from build123d import *

# Parameters (mm, degrees)
SALIENTE_EXTRUIR1_DEPTH = 155
CORTAR_EXTRUIR6_DEPTH   = 155
CROQUIS5_R              = 1.5
CORTAR_EXTRUIR9_DEPTH   = 155


with BuildPart() as part:
    # Croquis1 → Saliente-Extruir1 (new body)
    with BuildSketch(Plane.XY):
        with BuildLine():
            Line((0, 0), (28.5, 0))
            Line((28.5, 0), (0, 3))
            ThreePointArc((0, 3), (-1.5, 1.5), (0, 0))
        make_face()
    extrude(amount=-SALIENTE_EXTRUIR1_DEPTH)

    # Croquis3 → Cortar-Extruir6 (cut)
    with BuildSketch(Plane(origin=(0, 0, 0), x_dir=(1, 0, 0), z_dir=(0, 1, 0))):
        Polygon((28.5, 0), (28.5, 117.287187079), (16.5, 0), align=None)
        with BuildLine():
            ThreePointArc((7.5, 155), (11.035533906, 153.535533906), (12.5, 150))
            Line((12.5, 150), (12.5, 145))
            Line((12.5, 145), (28.5, 117.287187079))
            Line((28.5, 117.287187079), (28.5, 155))
            Line((28.5, 155), (7.5, 155))
        make_face()
        with BuildLine():
            ThreePointArc((3.5, 155), (-0.035533906, 153.535533906), (-1.5, 150))
            Line((-1.5, 150), (-1.5, 155))
            Line((-1.5, 155), (3.5, 155))
        make_face()
    extrude(amount=CORTAR_EXTRUIR6_DEPTH, mode=Mode.SUBTRACT)

    # Croquis5 → Cortar-Extruir9 (cut)
    with BuildSketch(Plane(origin=(0.312328767, 2.967123288, 0), x_dir=(0.9945054529214061, -0.10468478451804268, 0), z_dir=(0.10468478451804267, 0.994505452921406, 0))):
        with Locations(Location((5.255006945, 150, 0), (0, 0, 180))):
            Circle(CROQUIS5_R)
    extrude(amount=-CORTAR_EXTRUIR9_DEPTH, mode=Mode.SUBTRACT)


solid = part.part
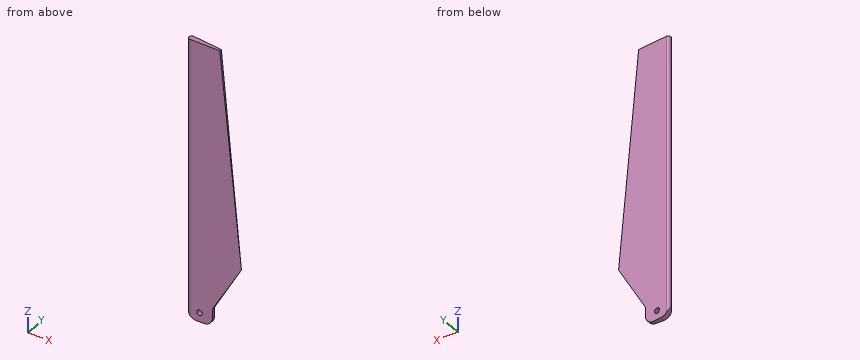
The model under review builds one solid part; all positions refer to its coordinate system, in mm. Round coordinates to 2 decimals unless told otherwise and drop trailing zeros. Write each loop counter-clockwise with the first axis right and the second up, starting at its lowest first coordinate (ties: lowest second). Pieces come first, ordered by that corner, then holes. Notation, with made-up numbers: (29.5, 27.5) - (78.5, 27.5) arc R24 cw to (78.5, 40.5) - close; hole circle Ø6 at (79.5, -40). An arc over 180 degrees is marked (long way). One line per item, written item: value. Start each with the question number.
1. Consider section A-A on x = 23. Write out the cut boundary in (y, z).
2. Clearance check with flat-ended pins moving along their axes: P1, Ø0.5, axis at y = 1, z = -148, coming from the +X side; P2, Ø2, axis at x = 6.5, z = -79, coming from the +Y side. State where each tip first meets the part, or that it passes through.
3. To check wall thickness, follow L1, parallel to Y at x = 12.5, z = -63.5; L2, parallel to Y at x = 4, z = -23; L3, parallel to Z at x = 1.5, y = 0.5. State the ranges of each line that lie inside material, in increasing order. Write a range as from..to.
4. Consider section B-B on z = -14.5. Write out the cut boundary in (x, y), and give its area (3 significant figures).
Checks:
1. outline: (0, -126.81) - (0.58, -126.81) - (0.58, -63.53) - (0, -63.53) - close
2. P1: stops at x = 12.5
2. P2: stops at y = 2.42
3. L1: y = 0..1.68
3. L2: y = 0..2.58
3. L3: z = -154.58..0
4. outline: (0, 0) - (17.98, 0) - (17.98, 1.11) - (0, 3) arc R1.5 ccw to start
4. area: 40.5 mm^2
